For this review, take the finished solid that the model builds, in its own axes (mm). A direction names the side the tool comes from. Round coordinates to 2 decimals unless told otherwise and drop trailing zeros. Loops run counter-clockwise (first coordinate to the right, second up) from the corner with the lowest first, then second, coordinate; pieces in that order, holes last. Notation, with made-up numbers: (8, -27.75) -> (18, -27.75) arc R10 ccw to (18, -21.75) -> close; hole circle Ø6 at (69, 62). An arc over 180 degrees is marked (long way). Use one line per item in the form item = value. Start each with the question number.
Autodesk Inventor part; units mm, degrees
ref_plane "Work Plane1" through (0, 0, 50) normal (0, 0, 1) x (1, 0, 0)
ref_plane "YZ Plane" through (0, 0, 0) normal (1, 0, 0) x (0, 1, 0)
ref_plane "XZ Plane" through (0, 0, 0) normal (0, 1, 0) x (-1, 0, 0)
sketch "Sketch1" plane through (0, 0, 0) normal (0, 0, 1) x (1, 0, 0)
  line L0 (0, -10) -> (0, 10)
  line L1 (10, 0) -> (-10, 0)
  line L2 (225, 175) -> (250, 175)
  line L3 (250, 175) -> (250, 200)
  line L4 (250, 200) -> (225, 200)
  line L5 (225, 200) -> (225, 175)
  line L6 (-225, 175) -> (-250, 175)
  line L7 (-250, 175) -> (-250, 200)
  line L8 (-250, 200) -> (-225, 200)
  line L9 (-225, 200) -> (-225, 175)
  line L10 (225, -175) -> (250, -175)
  line L11 (250, -175) -> (250, -200)
  line L12 (250, -200) -> (225, -200)
  line L13 (225, -200) -> (225, -175)
  line L14 (-225, -200) -> (-225, -175)
  line L15 (-250, -200) -> (-225, -200)
  line L16 (-250, -175) -> (-250, -200)
  line L17 (-225, -175) -> (-250, -175)
  point P0 (0, 0)
  dimension "d0" = 20
  dimension "d1" = 20
  dimension "d2" = 25
  dimension "d3" = 25
  dimension "d4" = 500
  dimension "d5" = 400
extrude "Extrusion1" add sketch "Sketch1" along normal blind 420
ref_plane "Work Plane1" through (0, 0, 50) normal (0, 0, 1) x (1, 0, 0)
sketch "Sketch6" plane through (0, 0, 50) normal (0, 0, 1) x (1, 0, 0)
  line L0 (-250, -175) -> (-250, -200)
  line L1 (250, 175) -> (250, 200)
  line L2 (-250, -200) -> (250, -200)
  line L3 (250, -200) -> (250, 200)
  line L4 (250, 200) -> (-250, 200)
  line L5 (-250, 200) -> (-250, -200)
  point P0 (0, 0)
extrude "Extrusion6" add sketch "Sketch6" against normal blind 5
sketch "Sketch7" plane through (0, 0, 45) normal (0, 0, -1) x (-1, 0, 0)
  line L0 (250, -200) -> (225, -200)
  line L1 (-250, 200) -> (-225, 200)
  line L2 (250, -200) -> (-250, -200)
  line L3 (-250, -200) -> (-250, 200)
  line L4 (-250, 200) -> (250, 200)
  line L5 (250, 200) -> (250, -200)
  line L6 (225, -175) -> (250, -175)
  line L7 (-225, 175) -> (-225, 200)
  line L8 (225, -175) -> (-225, -175)
  line L9 (-225, -175) -> (-225, 175)
  line L10 (-225, 175) -> (225, 175)
  line L11 (225, 175) -> (225, -175)
  point P0 (0, 0)
extrude "Extrusion7" add sketch "Sketch7" along normal blind 10 contours L0 L2 L3 L1 L7 L9 L8 L6 L5 | L6 L11 L10 L7 L4 L5
sketch "Sketch8" plane through (0, 0, 420) normal (0, 0, 1) x (1, 0, 0)
  line L0 (-225, 200) -> (-250, 200)
  line L1 (250, -200) -> (250, -175)
  line L2 (-250, 200) -> (250, 200)
  line L3 (250, 200) -> (250, -200)
  line L4 (250, -200) -> (-250, -200)
  line L5 (-250, -200) -> (-250, 200)
  line L6 (0, 150) -> (210, 150)
  line L7 (210, 150) -> (210, -150)
  line L8 (210, -150) -> (0, -150)
  line L9 (0, -150) -> (0, 150)
  point P0 (0, 0)
  dimension "d26" = 50
  dimension "d29" = 40
  dimension "d30" = 50
  dimension "d31" = 210
  dimension "d32" = 300
extrude "Extrusion8" add sketch "Sketch8" against normal blind 5
sketch "Sketch9" plane through (0, 0, 415) normal (0, 0, -1) x (-1, 0, 0)
  line L0 (250, -175) -> (250, -200)
  line L1 (-250, 200) -> (-225, 200)
  line L2 (250, -200) -> (-250, -200)
  line L3 (-250, -200) -> (-250, 200)
  line L4 (-250, 200) -> (250, 200)
  line L5 (250, 200) -> (250, -200)
  line L6 (225, -175) -> (250, -175)
  line L7 (-250, 175) -> (-225, 175)
  line L8 (225, -175) -> (-225, -175)
  line L9 (-225, -175) -> (-225, 175)
  line L10 (-225, 175) -> (225, 175)
  line L11 (225, 175) -> (225, -175)
  point P0 (0, 0)
extrude "Extrusion9" add sketch "Sketch9" along normal blind 10 contours L6 L11 L10 L7 L3 L1 L4 L5 | L0 L2 L3 L7 L9 L8 L6
equation "\"d30\" = d26"
properties part number "Table"
Item 1: Take a section at A-A on z = 276. Give the boundary of the cut face in (x, y), plus the area to 3 significant figures.
Item 2: Machinability: for faces 1 (the flat face through (-237, 175, 225)), 2 (the flat face through (-237, -175, 17)), 3 (the flat face through (-225, 188, 17)), which of the approach directions +Z, -Z, +X, -X, +Y, -Y give a long, thin tool a straight path to every point of the face, cutting with its end or side? Answer none if there is none.
Item 3: Take a section at C-C on y = -77.5. Give the boundary of the cut face in (x, z), plus the area to 3 significant figures.
Item 4: For P1, Ø12.5, axis at x = -233.5, y = -84.5, coming from the -Z side, flat-tipped, find the tip position at first contact; note if it passes through.
Item 5: Take a section at B-B on x = 38.5. Give the boundary of the cut face in (y, z), plus the area to 3 significant figures.
Item 6: Wall thickness on line 1 (Z direction, x = -96, y = 75.5); line 2 (X direction, y = 177, z = 200); line 3 (Z direction, x = 189, y = 36.5): over which ranges is each line inside the solid? List them lowest first.
Item 7: Draft analysis for pull direction X (two halves, no side actions). For faces 4 (the flat face through (250, 179, 227)), 5 (the flat face through (225, 188, 225)), 6 (the flat face through (237, -187, 0)), 7 (the flat face through (225, 188, 17)), state which applies: +X half, -X half, draft (parallel to the pull), parting line (faces both ways), or undercut.
Item 8: Take a section at D-D on y = 160.5. Give the boundary of the cut face in (x, z).
Results:
q1.outline = (-250, -200) -> (-225, -200) -> (-225, -175) -> (-250, -175) -> close; (-250, 175) -> (-225, 175) -> (-225, 200) -> (-250, 200) -> close; (225, -200) -> (250, -200) -> (250, -175) -> (225, -175) -> close; (225, 175) -> (250, 175) -> (250, 200) -> (225, 200) -> close
q1.area = 2,500 mm2
q2.face_1 = +X, -X
q2.face_2 = -Z, +X, -X
q2.face_3 = -Z, +Y, -Y
q3.outline = (-250, 35) -> (-225, 35) -> (-225, 45) -> (225, 45) -> (225, 35) -> (250, 35) -> (250, 50) -> (-250, 50) -> close; (-250, 405) -> (-225, 405) -> (-225, 415) -> (0, 415) -> (0, 420) -> (-250, 420) -> close; (210, 415) -> (225, 415) -> (225, 405) -> (250, 405) -> (250, 420) -> (210, 420) -> close
q3.area = 4,950 mm2
q4.P1 = 35
q5.outline = (-200, 35) -> (-175, 35) -> (-175, 45) -> (175, 45) -> (175, 35) -> (200, 35) -> (200, 50) -> (-200, 50) -> close; (-200, 405) -> (-175, 405) -> (-175, 415) -> (-150, 415) -> (-150, 420) -> (-200, 420) -> close; (150, 415) -> (175, 415) -> (175, 405) -> (200, 405) -> (200, 420) -> (150, 420) -> close
q5.area = 3,500 mm2
q6.line_1 = 45 to 50, 415 to 420
q6.line_2 = -250 to -225, 225 to 250
q6.line_3 = 45 to 50
q7.face_4 = +X half
q7.face_5 = undercut
q7.face_6 = draft
q7.face_7 = undercut
q8.outline = (-250, 35) -> (-225, 35) -> (-225, 45) -> (225, 45) -> (225, 35) -> (250, 35) -> (250, 50) -> (-250, 50) -> close; (-250, 405) -> (-225, 405) -> (-225, 415) -> (225, 415) -> (225, 405) -> (250, 405) -> (250, 420) -> (-250, 420) -> close
